Solid Edge part; units mm, degrees
sketch "Sketch1" plane through (0, 0, 0) normal (0, -1, 0) x (1, 0, 0)
  line L0 (1.5875, -36.478) -> (1.5875, -38.0669)
  arc A0 (1.5875, 38.0669) -> (1.5875, -38.0669) centre (0, 0) cw
  line L1 (1.5875, 38.0669) -> (1.5875, 36.478)
  arc A1 (1.5875, 36.478) -> (1.5875, -36.478) centre (0, 0) cw
extrude "Protrusion1" add sketch "Sketch1" along normal mid plane 127
sketch "Sketch2" plane through (0, 0, 0) normal (0, -1, 0) x (1, 0, 0)
  circle A0 centre (0, 49.1794) radius 6.35
  line L0 (1.5875, 38.0669) -> (1.5875, 41.2419)
  line L1 (1.5875, 41.2419) -> (0, 41.2419)
  line L2 (4.2974, 55.853) -> (26.9875, 41.2419)
  line L3 (26.9875, 41.2419) -> (26.9875, 26.894)
  arc A1 (26.9875, 26.894) -> (1.5875, 38.0669) centre (0, 0) ccw
  arc A2 (0, 41.2419) -> (4.2974, 55.853) centre (0, 49.1794) cw
  dimension "D1" = 1.5875
extrude "ExtrudedProtrusion_2" add sketch "Sketch2" along normal mid plane 76.2
sketch "Sketch3" plane through (0, 0, 0) normal (1, 0, 0) x (0, 1, 0)
  line L0 (-12.7, 41.2419) -> (12.7, 41.2419)
  line L1 (12.7, 57.1169) -> (12.7, 41.2419)
  line L2 (-12.7, 57.1169) -> (12.7, 57.1169)
  line L3 (-12.7, 57.1169) -> (-12.7, 41.2419)
extrude "ExtrudedCutout_1" cut sketch "Sketch3" along normal mid plane 118.5822
sketch "Sketch4" plane through (19.8438, -63.5, 0) normal (0, -1, 0) x (0, 0, -1)
  line L0 (-38.0669, -18.2562) -> (-38.0669, 16.089)
  line L1 (-12.6669, 16.089) -> (-38.0669, 16.089)
  line L2 (-12.6669, -18.2562) -> (-12.6669, 16.089)
  line L3 (-38.0669, -18.2562) -> (-12.6669, -18.2562)
extrude "ExtrudedCutout_2" cut sketch "Sketch4" against normal blind 3.302
Build history of the part. All positions in model axes, mm. A direction names the side the tool comes from. Give positions to 0.01 mm unless a question says otherwise; leave off trailing zeros. Loops run counter-clockwise (first coordinate to the right, second up) from the corner with the lowest first, then second, coordinate; pieces in that order, holes last.
Item 1: Slice it at C-C, the plane z = 0. List the corners of the cut face in (x, y).
Answers follow:
outline: (36.51, -63.5) - (38.1, -63.5) - (38.1, 63.5) - (36.51, 63.5) - close
Item 2: Which spindle directions (+Z, -Z, +X, -X, +Y, -Y) get a long thin tool onto all of the face, cutting with end or side? Do faces 4 (the face through (14, -38.1, 42)), 5 (the face through (23, -60.198, 29)), 6 (the face through (14, 0, 41.242)), 7 (the face through (36.504, 0.889, 0.781)). Say none if no direction does.
Answers follow:
face 4: +Z, +X, -Y
face 5: +Z, +X, -X, -Y
face 6: +Z, +X, -X
face 7: -X, +Y, -Y
Item 3: Pull direction X, two halves, no side cores. Call faces 1 (the face through (14, 38.1, 42)), 2 (the face through (-0.827, -25.222, 42.883)), 3 (the face through (15.48, -25.22, 48.65)): released by +X, released by -X, zero draft, split by the parting line, or undercut.
Answers follow:
face 1: zero draft
face 2: undercut
face 3: released by +X
Item 4: Flat gauge pins, fed straight in: pin 1 (1.5 mm diameter, centred on x = 25.5, y = -15.5, fed in from +Z); pin 2 (0.8 mm diameter, centred on x = 35, y = -62.5, fed in from +Z); pin 3 (8 mm diameter, centred on x = 3, z = 53, fed in from -Y). Where does each tip first touch, or does it go through?
Answers follow:
pin 1: stops at z = 42.68
pin 2: stops at z = 12.67
pin 3: stops at y = -38.1
Item 5: Slice it at B-B, the plane x = 12.5. List the corners of the cut face in (y, z).
Answers follow:
outline: (-63.5, -35.99) - (63.5, -35.99) - (63.5, -34.31) - (-63.5, -34.31) - close; (-60.2, 34.31) - (63.5, 34.31) - (63.5, 35.99) - (38.1, 35.99) - (38.1, 50.57) - (12.7, 50.57) - (12.7, 41.24) - (-12.7, 41.24) - (-12.7, 50.57) - (-38.1, 50.57) - (-38.1, 35.99) - (-60.2, 35.99) - close
Item 6: Drill centre lines: line 1 (Z direction, x = 0, y = 18.75); line 2 (Z direction, x = 20.5, y = -40.5); line 3 (X direction, y = 22.5, z = 50). Where is each one in solid material? Low to high.
Answers follow:
line 1: z = 41.24 to 42.83, 55.53 to 57.12
line 2: z = -32.11 to -30.21, 30.21 to 32.11
line 3: x = -7.89 to -6.3, 6.3 to 13.39
